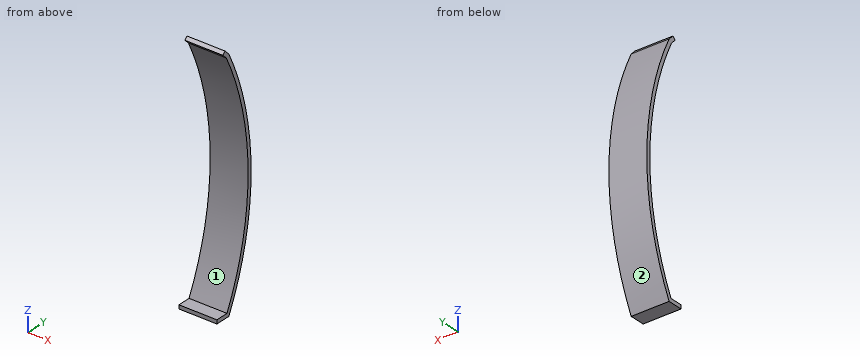
from build123d import *

# Parameters (mm, degrees)
F1_DEPTH = 5


with BuildPart() as f1:
    # F0 (on Right) → F1 (new body)
    with BuildSketch(Plane.YZ):
        with BuildLine():
            Line((0, 0.5), (0, 0))
            Line((0, 0), (2, 0))
            ThreePointArc((2, 0), (5.707211, 15.676777), (2, 31.353553))
            Line((2, 31.353553), (1.353553, 32))
            Line((1.353553, 32), (1, 31.646447))
            Line((1, 31.646447), (1.589002, 31.057444))
            ThreePointArc((1.589002, 31.057444), (5.207023, 15.79048), (1.689713, 0.5))
            Line((1.689713, 0.5), (0, 0.5))
        make_face()
    extrude(amount=F1_DEPTH)


solid = f1.part
Can you work these out from the model? Positions are in its coordinate system, mm. Face numbers are marked on the shaded views. Give positions to 0.01 mm unless a question says otherwise; leave off trailing zeros. Order: outer loops, then holes, each group sorted by start corner. A loop starts at its lowest first (then second) coordinate and runs counter-clockwise, first axis right, second up. Notation, with made-up numbers: M -4,29 L 11,29 A33 ccw 11,60 Z; hole C -8,-9 d5. An arc over 180 degrees is marked long. Use a Markdown table: item, result. Add a question column.
Item 1: We'd pull the mould along Z, two halves only. Please class the marked faces 1 and 2: +Z half, -Z half, draft (parallel to the pull), parting line (faces both ways), or undercut.
Item 2: If I drill on L1, parallel to Z at x = 3, y = 2.3; L2, parallel to Y at x = 1.25, z = 21; L3, parallel to Y at x = 4.3, z = 11, over which ranges is the centre line in solid material (lowest first)? Write a range as [from, to].
Item 3: Suppose I cut it at B-B (x = 3.1). List the corners of the cut face in (y, z) for me, then the cut area to 3 significant figures.
Item 4: Will these pins go through, and if not, where does the flat tip stop? pin 1 (3 mm diameter, centred on x = 3, z = 19, fed in from +Y); pin 2 (1.5 mm diameter, centred on x = 2.5, z = 12, fed in from +Y); pin 3 (1 mm diameter, centred on x = 2, z = 5, fed in from +Y) (3 decimals); pin 4 (1.9 mm diameter, centred on x = 1.5, y = 0.5, fed in from +Z).
Item 5: Suppose I cut it at A-A (y = 4.45). List the corners of the cut face in (x, z) for me.
Item 6: Suppose I cut it at C-C (y = 0.6). List the corners of the cut face in (x, z) for me.
Item 7: Suppose I cut it at D-D (z = 29). List the corners of the cut face in (x, y) for me, then the cut area to 3 significant figures.
Answer sheet:
| question | item | result |
|---|---|---|
| 1 | face 1 | undercut |
| 1 | face 2 | parting line |
| 2 | L1 | z = [0.61, 1.82], [29.54, 30.74] |
| 2 | L2 | y = [4.79, 5.3] |
| 2 | L3 | y = [4.89, 5.39] |
| 3 | outline | M 0,0 L 2,0 A35 ccw 2,31.35 L 1.35,32 L 1,31.65 L 1.59,31.06 A34.5 cw 1.69,0.5 L 0,0.5 Z |
| 3 | area | 17.4 mm² |
| 4 | pin 1 | stops at y = 5.66 |
| 4 | pin 2 | stops at y = 5.58 |
| 4 | pin 3 | stops at y = 4.195 |
| 4 | pin 4 | stops at z = 32 |
| 5 | outline | M 0,6.38 L 5,6.38 L 5,8.49 L 0,8.49 Z; M 0,22.87 L 5,22.87 L 5,24.97 L 0,24.97 Z |
| 6 | outline | M 0,0 L 5,0 L 5,0.5 L 0,0.5 Z |
| 7 | outline | M 0,2.53 L 5,2.53 L 5,3.07 L 0,3.07 Z |
| 7 | area | 2.71 mm² |
